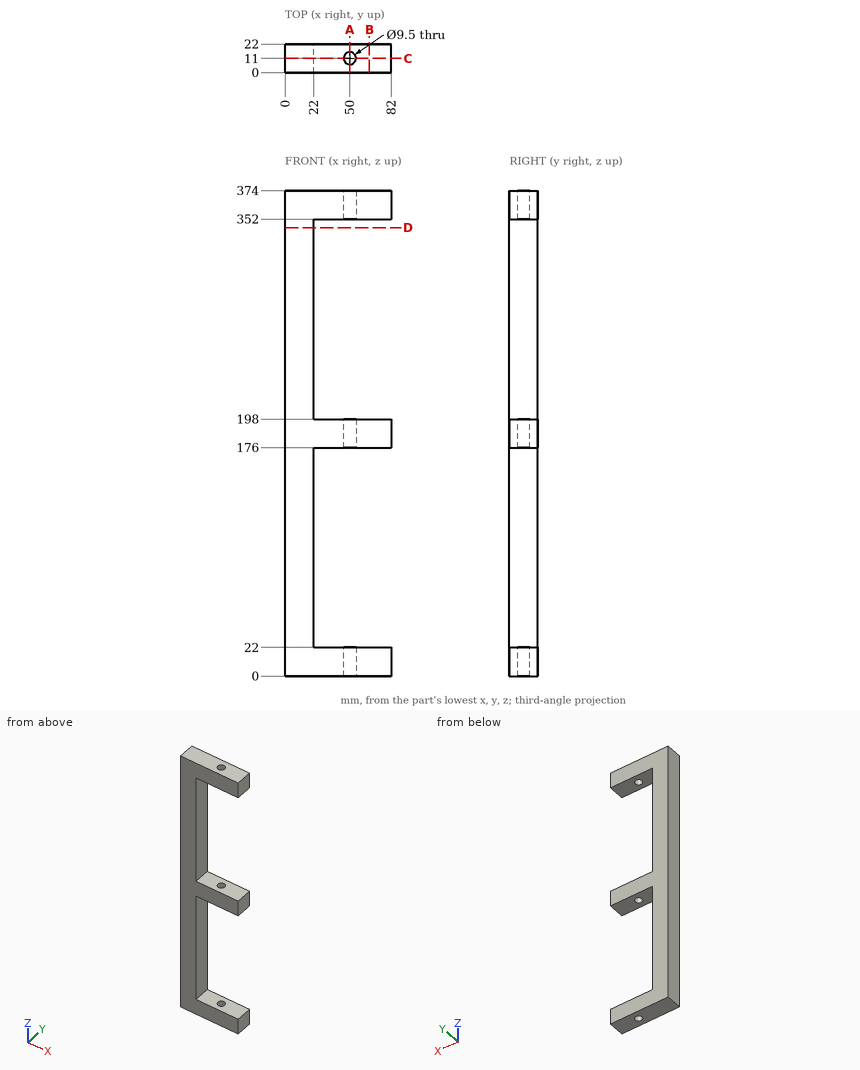
The figure shows three views and two pictorial views of one solid part (mm, origin at its lowest corner). Answer the questions. Coordinates: 2 decimals unless noted, no trailing zeros. Loops run counter-clockwise (first coordinate to the right, second up) from the corner with the lowest first, then second, coordinate; pieces in that order, holes last. Notation, with made-up numbers: (77, -35) - (126, -35) arc R20 ccw to (126, 4) - close; hole circle Ø3 at (-22, 56). An arc over 180 degrees is marked (long way). Answer in a Markdown table with one row per item.
Q1. Find section B-B on x = 65. Write down the section's boundary in (y, z), plus the area to 3 significant figures.
Here are the results:
| item | result |
|---|---|
| outline | (0, 0) - (22, 0) - (22, 22) - (0, 22) - close; (0, 176) - (22, 176) - (22, 198) - (0, 198) - close; (0, 352) - (22, 352) - (22, 374) - (0, 374) - close |
| area | 1,450 mm^2 |
Q2. Straight lines are drawn through the part: line 1 along Z through (x, y) = (63.5, 16.25); line 2 along Y through (x, z) = (50, 360); line 3 along X through (y, z) = (13, 302.5). For each, find the intervals that lie inside material, in ascending order. Write a range as [from, to].
Here are the results:
| item | result |
|---|---|
| line 1 | z = [0, 22], [176, 198], [352, 374] |
| line 2 | y = [0, 6.25], [15.75, 22] |
| line 3 | x = [0, 22] |
Q3. Find section D-D on z = 345.5. Write down the section's boundary in (x, y).
Here are the results:
| item | result |
|---|---|
| outline | (0, 0) - (22, 0) - (22, 22) - (0, 22) - close |
Q4. Given P1, Ø6.5, axis at y = 5.5, z = 312, coming from the +X side; P2, Ø5.5, axis at x = 50, y = 11, coming from the +Z side, each flat-ended and moving along its own axis, determine where each tip first touches the part or whether it passes through.
Here are the results:
| item | result |
|---|---|
| P1 | stops at x = 22 |
| P2 | passes through |
Q5. Find section C-C on y = 11. Write down the section's boundary in (x, z), plus the area to 3 significant figures.
Here are the results:
| item | result |
|---|---|
| outline | (0, 0) - (45.25, 0) - (45.25, 22) - (22, 22) - (22, 176) - (45.25, 176) - (45.25, 198) - (22, 198) - (22, 352) - (45.25, 352) - (45.25, 374) - (0, 374) - close; (54.75, 0) - (82, 0) - (82, 22) - (54.75, 22) - close; (54.75, 176) - (82, 176) - (82, 198) - (54.75, 198) - close; (54.75, 352) - (82, 352) - (82, 374) - (54.75, 374) - close |
| area | 11,600 mm^2 |
Q6. Find section A-A on x = 50. Write down the section's boundary in (y, z), plus the area to 3 significant figures.
Here are the results:
| item | result |
|---|---|
| outline | (0, 0) - (6.25, 0) - (6.25, 22) - (0, 22) - close; (0, 176) - (6.25, 176) - (6.25, 198) - (0, 198) - close; (0, 352) - (6.25, 352) - (6.25, 374) - (0, 374) - close; (15.75, 0) - (22, 0) - (22, 22) - (15.75, 22) - close; (15.75, 176) - (22, 176) - (22, 198) - (15.75, 198) - close; (15.75, 352) - (22, 352) - (22, 374) - (15.75, 374) - close |
| area | 825 mm^2 |
